Autodesk Inventor part; units mm, degrees
ref_plane "YZ Plane" through (0, 0, 0) normal (1, 0, 0) x (0, 1, 0)
ref_plane "XZ Plane" through (0, 0, 0) normal (0, 1, 0) x (-1, 0, 0)
ref_plane "XY Plane" through (0, 0, 0) normal (0, 0, 1) x (1, 0, 0)
sketch "Skizze1" plane through (0, 0, 0) normal (0, 0, 1) x (1, 0, 0)
  circle A0 centre (0, 0) radius 26
  dimension "d0" = 52
extrude "Extrusion1" add sketch "Skizze1" along normal blind 19
hole "Bohrung1" at (0, 0, 19) direction (0, 0, -1) diameter 35 depth 20 counterbore diameter 38.3 counterbore depth 17
sketch "Skizze2" plane through (0, 0, 19) normal (0, 0, 1) x (1, 0, 0)
  circle A0 centre (0, -22.5) radius 2.525
  point P0 (0, 0)
  dimension "d12" = 5.05
  dimension "d13" = 22.5
extrude "Extrusion2" cut sketch "Skizze2" against normal blind 2.1
pattern_circular "Runde Anordnung1" count 3 over 360 about axis through (0, 0, 0) along (0, 0, 1) of "Extrusion2"
properties part number "Sensor Deckel383"
Here's how the part is built. I have some questions about the finished solid (model axes, mm). A direction names the side the tool comes from. Coordinates: 2 decimals unless noted, no trailing zeros. Order: outer loops, then holes, each group sorted by start corner. A loop starts at its lowest first (then second) coordinate and runs counter-clockwise, first axis right, second up.
Item 1: If we section it at D-D on y = -22.5: List the corners of the cut face in (x, z) for me (3 decimals), plus the area to 3 significant figures.
Result sheet:
outline: (-13.029, 0) - (13.029, 0) - (13.029, 19) - (2.525, 19) - (2.525, 16.9) - (-2.525, 16.9) - (-2.525, 19) - (-13.029, 19) - close
area: 484 mm2
Item 2: If we mould it in two halves opening along X, with no side actions, what happens to faces 3 (the face through (16, -8, 2)), 4 (the face through (-20.633, 15.821, 9.367)), 5 (the face through (5, -17, 0)), 6 (the face through (17.625, 12.957, 17.965))? For each: +X half, -X half, draft (parallel to the pull), parting line (faces both ways), or undercut.
Result sheet:
face 3: undercut
face 4: parting line
face 5: draft
face 6: undercut
Item 3: If we section it at A-A on y = 0: List the corners of the cut face in (x, z) for me, plus the area to 3 significant figures.
Result sheet:
outline: (-26, 0) - (-17.5, 0) - (-17.5, 2) - (-19.15, 2) - (-19.15, 19) - (-26, 19) - close; (17.5, 0) - (26, 0) - (26, 19) - (19.15, 19) - (19.15, 2) - (17.5, 2) - close
area: 267 mm2
Item 4: For P1, Ø2, axis at y = -9, z = 14.5, coming from the -X side; P2, Ø6.5, axis at x = 0, y = -22.5, coming from the +Z side; P3, Ø4, axis at x = -20, z = 11.5, coming from the -Y side; P4, Ø4, axis at y = 5, z = 13.5, coming from the +X side, each with a flat end and sliding along its axis, tell me the tip position at first contact or that it passes through.
Result sheet:
P1: stops at x = -24.74
P2: stops at z = 19
P3: stops at y = -18.76
P4: stops at x = 25.83
Item 5: I need wall thicknesses on line 1 (Y direction, x = 0, z = 18.2) (3 decimals); line 2 (X direction, y = -0.5, z = 5.5); line 3 (Y direction, x = 5.5, z = 17). Which ranges of each line are inside material? Lowest first, please.
Result sheet:
line 1: y = -26 to -25.025, -19.975 to -19.15, 19.15 to 26
line 2: x = -26 to -19.14, 19.14 to 26
line 3: y = -25.41 to -18.34, 18.34 to 25.41
Item 6: If we section it at B-B on x = 11: List the corners of the cut face in (y, z) for me.
Result sheet:
outline: (-23.56, 0) - (-13.61, 0) - (-13.61, 2) - (-15.68, 2) - (-15.68, 19) - (-23.56, 19) - close; (13.61, 0) - (23.56, 0) - (23.56, 19) - (15.68, 19) - (15.68, 2) - (13.61, 2) - close
Item 7: If we section it at C-C on z = 7: List the corners of the cut face in (x, y) for me.
Result sheet:
outline: circle Ø52 at (0, 0); hole circle Ø38.3 at (0, 0)
Item 8: For faces 1 (the face through (10.648, 13.887, 0.986)), 2 (the face through (19, 11, 16.9)), which set-ups out of +Z, -Z, +X, -X, +Y, -Y let a thin tool reach every point of the face, with its end or its side?
Result sheet:
face 1: +Z, -Z
face 2: +Z
